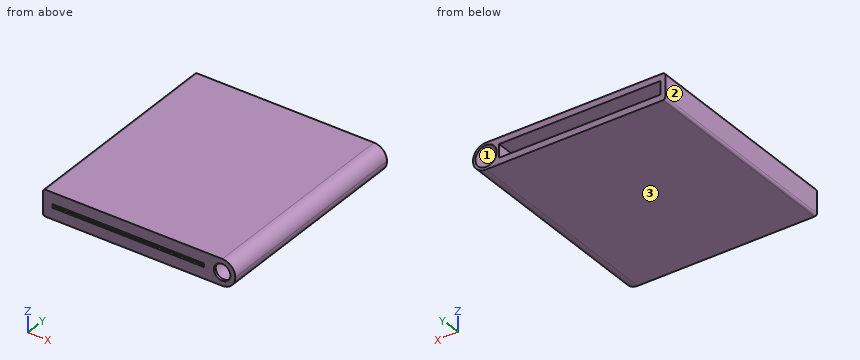
```python
from build123d import *

# Parameters (mm, degrees)
SKETCH_W     = 126.4
SKETCH_H     = 17.2
SKETCH_R     = 7
SKETCH_W_2   = 106
SKETCH_H_2   = 8.75
PAD_DEPTH    = 138
SKETCH001_W  = 126.4
SKETCH001_H  = 17.2
SKETCH001_R  = 5.4
PAD001_DEPTH = 1.6
FILLET_R     = 8.5
FILLET001_R  = 1.6
SKETCH002_W  = 99.6
SKETCH002_H  = 2.35
POCKET_DEPTH = 5


with BuildPart() as part:
    # Sketch → Pad (new body)
    with BuildSketch(Plane.XZ):
        with Locations((7, 0)):
            Rectangle(SKETCH_W, SKETCH_H)
        with Locations((61.6, 0)):
            Circle(SKETCH_R, mode=Mode.SUBTRACT)
        Rectangle(SKETCH_W_2, SKETCH_H_2, mode=Mode.SUBTRACT)
    extrude(amount=PAD_DEPTH)

    # Sketch001 (on Face11 of Pad) → Pad001 (join)
    with BuildSketch(Plane.XZ.offset(138)):
        with Locations((7, 0)):
            Rectangle(SKETCH001_W, SKETCH001_H)
        with Locations((61.6, 0)):
            Circle(SKETCH001_R, mode=Mode.SUBTRACT)
    extrude(amount=PAD001_DEPTH)

    # Fillet
    fillet_edges = [part.edges().sort_by_distance(p)[0] for p in [
        (70.2, -69.8, 8.6),
        (70.2, -69.8, -8.6),
    ]]
    fillet(fillet_edges, radius=FILLET_R)

    # Fillet001
    fillet001_edges = [part.edges().sort_by_distance(p)[0] for p in [
        (-56.2, -69.8, 8.6),
        (-56.2, -69.8, -8.6),
    ]]
    fillet(fillet001_edges, radius=FILLET001_R)

    # Sketch002 (on Face16 of Fillet001) → Pocket (cut)
    with BuildSketch(Plane(origin=(0, -138, 0), x_dir=(1, 0, 0), z_dir=(0, 1, 0))):
        Rectangle(SKETCH002_W, SKETCH002_H)
    extrude(amount=-POCKET_DEPTH, mode=Mode.SUBTRACT)


solid = part.part
```
Geometry check sheet. Reference: the model listing, model coordinates, mm. Face numbers are marked on the shaded views. Round coordinates to 2 decimals unless told otherwise and drop trailing zeros. Order: outer loops, then holes, each group sorted by start corner. A loop starts at its lowest first (then second) coordinate and runs counter-clockwise, first axis right, second up. Notation, with made-up numbers: (-20.5, 28) -> (-9.5, 28) arc R9 ccw to (-9.5, 41) -> close; hole circle Ø10 at (55.25, 26.5). An arc over 180 degrees is marked (long way). Return JSON: item names as keys, results as strings. Group by question number.
Q1. Section check D-D, the plane x = 58.5. Record the boundary of the cut face in (y, z).
Q2. Gauge pin test, flat ends, axial feed: pin 1 (1 mm diameter, centred on y = -45, z = -2, fed in from +X); pin 2 (1 mm diameter, centred on y = -81, z = -5, fed in from +X); pin 3 (3 mm diameter, centred on y = -92, z = 6.5, fed in from +X). Record the tip position at first contact, or that the pin passes through.
Q3. Section check C-C, the plane z = 2.75. Record the boundary of the cut face in (x, y).
Q4. Section check B-B, the plane y = -91. Record the boundary of the cut face in (x, z) (3 decimals).
Q5. Release check for a two-part mould opening along X. For the marked faces 1, 2 and 3 record: released by +X, released by -X, zero draft, split by the parting line, or undercut.
Q6. Section check A-A, the plane x = -20. Record the boundary of the cut face in (y, z) (3 decimals), plus the area to 3 significant figures.
Q7. Material ranges on probe 1 along Z at (x, y) = (23.5, -65.5) (3 decimals); probe 2 along Z at (x, y) = (61.6, -138.4); probe 3 along X at (y, z) = (-132, 2), recorded low to high. Write a range as from..to.
Numbers:
{
 "1": {"outline": "(-139.6, -8.6) -> (0, -8.6) -> (0, -6.28) -> (-138, -6.28) -> (-138, -4.42) -> (-139.6, -4.42) -> close; (-139.6, 4.42) -> (-138, 4.42) -> (-138, 6.28) -> (0, 6.28) -> (0, 8.6) -> (-139.6, 8.6) -> close"},
 "2": {"pin 1": "x = 70.08", "pin 2": "x = 68.97", "pin 3": "x = 68.65"},
 "3": {"outline": "(-56.2, -139.6) -> (56.95, -139.6) -> (56.95, -138) -> (55.16, -138) -> (55.16, 0) -> (53, 0) -> (53, -138) -> (-53, -138) -> (-53, 0) -> (-56.2, 0) -> close; (66.25, -139.6) -> (69.78, -139.6) -> (69.78, 0) -> (68.04, 0) -> (68.04, -138) -> (66.25, -138) -> close"},
 "4": {"outline": "(-56.2, -7) arc R1.6 ccw to (-54.6, -8.6) -> (61.7, -8.6) arc R8.5 ccw to (70.2, -0.1) -> (70.2, 0.1) arc R8.5 ccw to (61.7, 8.6) -> (-54.6, 8.6) arc R1.6 ccw to (-56.2, 7) -> close; hole (-53, -4.375) -> (53, -4.375) -> (53, 4.375) -> (-53, 4.375) -> close; hole circle Ø14 at (61.6, 0)"},
 "5": {"face 1": "undercut", "face 2": "released by -X", "face 3": "zero draft"},
 "6": {"outline": "(-139.6, -8.6) -> (0, -8.6) -> (0, -4.375) -> (-138, -4.375) -> (-138, -1.175) -> (-139.6, -1.175) -> close; (-139.6, 1.175) -> (-138, 1.175) -> (-138, 4.375) -> (0, 4.375) -> (0, 8.6) -> (-139.6, 8.6) -> close", "area": "1,190 mm^2"},
 "7": {"probe 1": "-8.6..-4.375, 4.375..8.6", "probe 2": "-8.6..-5.4, 5.4..8.6", "probe 3": "-56.2..-53, 53..54.89, 68.31..69.98"}
}
